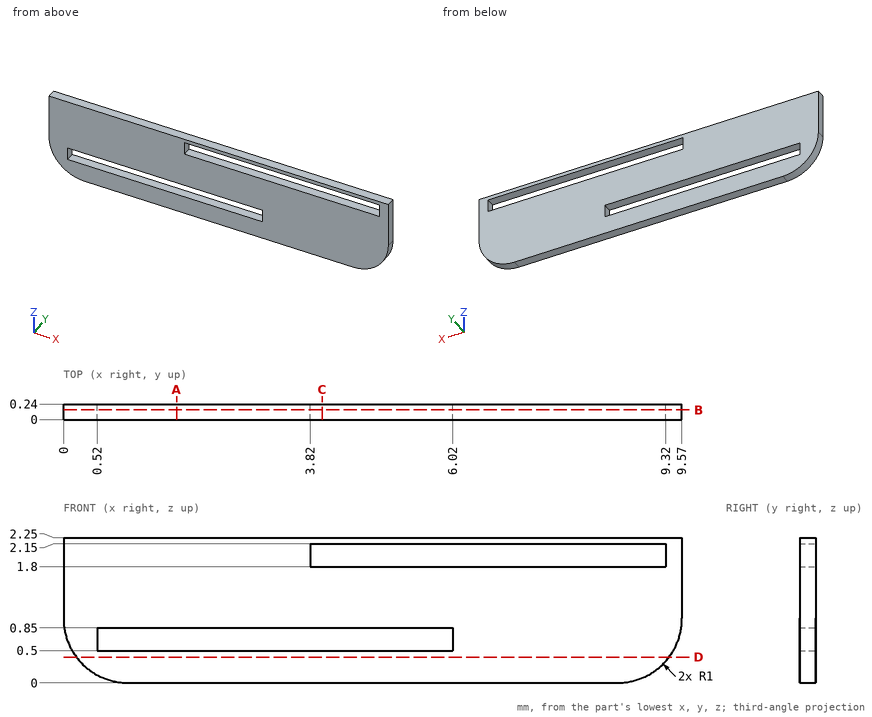
Here's the drawing with two shaded views (mm, measured from the low corner). I have some questions. Round coordinates to 2 decimals unless told otherwise and drop trailing zeros. Write each loop counter-clockwise with the first axis right and the second up, starting at its lowest first coordinate (ties: lowest second). Pieces come first, ordered by that corner, then holes.
(1) If I drill on probe 1 along Z at (x, y) = (2.75, 0.15); probe 2 along X at (y, z) = (0.15, 2); probe 3 along X at (y, z) = (0.15, 0.8), over which ranges is the centre line in solid material (lowest first)?
Findings below:
probe 1: z = 0 to 0.5, 0.85 to 2.25
probe 2: x = 0 to 3.82, 9.32 to 9.57
probe 3: x = 0.02 to 0.52, 6.02 to 9.55
(2) Suppose I cut it at A-A on x = 1.75. Write out the boundary of the cut face in (y, z), and give its area (3 significant figures).
Findings below:
outline: (0, 0) - (0.24, 0) - (0.24, 0.5) - (0, 0.5) - close; (0, 0.85) - (0.24, 0.85) - (0.24, 2.25) - (0, 2.25) - close
area: 0.456 mm2
(3) Suppose I cut it at C-C on x = 4. Write out the boundary of the cut face in (y, z), and give its area (3 significant figures).
Findings below:
outline: (0, 0) - (0.24, 0) - (0.24, 0.5) - (0, 0.5) - close; (0, 0.85) - (0.24, 0.85) - (0.24, 1.8) - (0, 1.8) - close; (0, 2.15) - (0.24, 2.15) - (0.24, 2.25) - (0, 2.25) - close
area: 0.372 mm2
(4) Suppose I cut it at B-B on y = 0.15. Write out the boundary of the cut face in (x, z).
Findings below:
outline: (0, 1) arc R1 ccw to (1, 0) - (8.57, 0) arc R1 ccw to (9.57, 1) - (9.57, 2.25) - (0, 2.25) - close; hole (0.52, 0.5) - (6.02, 0.5) - (6.02, 0.85) - (0.52, 0.85) - close; hole (3.82, 1.8) - (9.32, 1.8) - (9.32, 2.15) - (3.82, 2.15) - close
(5) Suppose I cut it at D-D on z = 0.4. Write out the boundary of the cut face in (x, y).
Findings below:
outline: (0.2, 0) - (9.37, 0) - (9.37, 0.24) - (0.2, 0.24) - close
